CAD build for the part. Positions are in the model's coordinates, mm. Coordinates: 2 decimals unless noted, no trailing zeros. Loops run counter-clockwise (first coordinate to the right, second up) from the corner with the lowest first, then second, coordinate; pieces in that order, holes last. Notation, with made-up numbers: (5, 59.25) - (13, 59.25) arc R24 ccw to (13, 69.25) - close; hole circle Ø11 at (32, 49.5). An arc over 180 degrees is marked (long way). Put each result on its own line as item: value.
```python
from build123d import *

# Parameters (mm, degrees)
EXTRUDE_1_DEPTH     = 40
FILLET_1_R          = 2
CHAMFER_2_SIZE      = 0.5
SKETCH_2_R          = 1.25
CUT_EXTRUDE_1_DEPTH = 44.772367073


with BuildPart() as part:
    # 草图1 → 凸台-拉伸1 (new body)
    with BuildSketch(Plane(origin=(0, 0, 0), x_dir=(0, 0, -1), z_dir=(1, 0, 0))):
        Polygon((0, 0), (15, 5.459553514), (15, -9.540446486), (0, -9.540446486), align=None)
    extrude(amount=-EXTRUDE_1_DEPTH)

    # 圆角1
    fillet_1_edges = [part.edges().sort_by_distance(p)[0] for p in [
        (-20, -9.540446486, 0),
    ]]
    fillet(fillet_1_edges, radius=FILLET_1_R)

    # 倒角2
    chamfer_2_edges = [part.edges().sort_by_distance(p)[0] for p in [
        (-20, -9.540446486, -15),
    ]]
    chamfer(chamfer_2_edges, length=CHAMFER_2_SIZE)

    # 草图2 → 切除-拉伸1 (cut, through all)
    with BuildSketch(Plane(origin=(0, 0, -15), x_dir=(-1, 0, 0), z_dir=(0, 0, -1))):
        with Locations((20, 0.459553514)):
            Circle(SKETCH_2_R)
        with Locations((27.5, 0.459553514)):
            Circle(SKETCH_2_R)
        with Locations((12.5, 0.459553514)):
            Circle(SKETCH_2_R)
        with Locations((20, -7.040446486)):
            Circle(SKETCH_2_R)
    extrude(amount=-CUT_EXTRUDE_1_DEPTH, mode=Mode.SUBTRACT)


solid = part.part
```
Q1. Slice it at C-C, the plane z = -10. Give the cut face in (x, y), then the cut area to 3 significant figures.
Determined:
outline: (-40, -9.54) - (0, -9.54) - (0, 3.64) - (-40, 3.64) - close; hole circle Ø2.5 at (-27.5, 0.46); hole circle Ø2.5 at (-20, -7.04); hole circle Ø2.5 at (-20, 0.46); hole circle Ø2.5 at (-12.5, 0.46)
area: 508 mm2
Q2. Slice it at B-B, the plane x = -20. Give the cut face in (y, z).
Determined:
outline: (-9.54, -14.5) - (-9.04, -15) - (-8.29, -15) - (-8.29, -0.15) arc R2 ccw to (-9.54, -2) - close; (-5.79, -15) - (-0.79, -15) - (-0.79, 0) - (-5.79, 0) - close; (1.71, -15) - (5.46, -15) - (1.71, -4.7) - close
Q3. Slice it at A-A, the plane x = -12.5. Give the cut face in (y, z), then the cut area to 3 significant figures.
Determined:
outline: (-9.54, -14.5) - (-9.04, -15) - (-0.79, -15) - (-0.79, 0) - (-7.54, 0) arc R2 ccw to (-9.54, -2) - close; (1.71, -15) - (5.46, -15) - (1.71, -4.7) - close
area: 150 mm2
Q4. Mould opens along Y. For faces 1 (the flat face through (-20, -9.54, -8)), 2 (the flat face through (-20, -4, 0)), 3 (the cylindrical face through (-28.077, -0.649, -7.605)) say: +Y half, -Y half, draft (parallel to the pull), parting line (faces both ways), or undercut.
Determined:
face 1: -Y half
face 2: draft
face 3: undercut
Q5. Wall check: L1, parallel to Y at x = -20, z = -9.75; L2, parallel to X at y = 1.5, z = -4.5; L3, parallel to Y at x = -19, z = -9.5. Give the ranges that are in metal, low to high. Write a range as from..to.
Determined:
L1: -9.54..-8.29, -5.79..-0.79, 1.71..3.55
L2: -40..-28.19, -26.81..-20.69, -19.31..-13.19, -11.81..0
L3: -9.54..-7.79, -6.29..-0.29, 1.21..3.46
